```python
from build123d import *

# Parameters (mm, degrees)
SKETCH1_R             = 2
BOSS_EXTRUDE1_DEPTH   = 15
BOSS_EXTRUDE1_2_DEPTH = 15
SKETCH2_W             = 34.599574116
SKETCH2_H             = 26.046082642
BOSS_EXTRUDE2_DEPTH   = 2


with BuildPart() as part:
    # Sketch1 → Boss-Extrude1 (new body)
    with BuildSketch(Plane.XY):
        Circle(SKETCH1_R)
    extrude(amount=BOSS_EXTRUDE1_DEPTH)



with BuildPart() as body_2:
    # Sketch1 → Boss-Extrude1 2 (new body)
    with BuildSketch(Plane.XY):
        with Locations((28.8, -20.2)):
            Circle(SKETCH1_R)
    extrude(amount=BOSS_EXTRUDE1_2_DEPTH)


with BuildPart() as part_1:
    add(part.part)

    add(body_2.part)  # Boss-Extrude2 merges body 2
    # Sketch2 → Boss-Extrude2 (add)
    with BuildSketch(Plane.XY):
        with Locations((14.329889414, -10.310331758)):
            Rectangle(SKETCH2_W, SKETCH2_H)
    extrude(amount=-BOSS_EXTRUDE2_DEPTH)


solid = part_1.part
```
Source: CAD feature listing. Evaluate the final solid. Frame: model axes, mm. A direction names the side the tool comes from. Give positions to 0.01 mm unless a question says otherwise; leave off trailing zeros. Loops run counter-clockwise (first coordinate to the right, second up) from the corner with the lowest first, then second, coordinate; pieces in that order, holes last. Notation, with made-up numbers: (-23, -1.75) -> (3, -1.75) arc R18 cw to (3, 28.25) -> close; hole circle Ø5 at (66, -1.75). An arc over 180 degrees is marked (long way). Use a Markdown table: item, result. Add a question column.
(1) Access query for faces 1 (the face through (0, 0, 15)), 2 (the face through (26.802, -20.112, 7.395)). Directions: +Z, -Z, +X, -X, +Y, -Y. A direction counts if a zero-diameter tool reaches every point of the face in a straight line with its end or side. Return the directions, or none.
(2) Section query B-B (x = 28.8). Output: boundary loops of the cut face in (y, z), then the cut area to 3 significant figures.
(3) First-contact query: pin 1 Ø8 at (y, z) = (-2.5, 2.5) entering from +X; pin 2 Ø8 at (x, y) = (14.5, -6) entering from +Z. Flat tips, straight axial feed; report the tip coordinate or a pass-through.
(4) Ray query, line 1 (Z direction, x = 2, y = -2); line 2 (Y direction, x = 0, z = 13.5); line 3 (X direction, y = -19.5, z = 11). Return the intervals inside material, ascending.
(5) Section query C-C (z = 11.75). Output: boundary loops of the cut face in (x, y), then the cut area to 3 significant figures.
(6) Section query D-D (y = -4.25). Output: boundary loops of the cut face in (x, z), then the cut area to 3 significant figures.
(7) Section query A-A (y = -20.2). Output: boundary loops of the cut face in (x, z).
Checked values:
| question | item | result |
|---|---|---|
| 1 | face 1 | +Z, +X, -X, +Y, -Y |
| 1 | face 2 | +Z |
| 2 | outline | (-23.33, -2) -> (2.71, -2) -> (2.71, 0) -> (-18.2, 0) -> (-18.2, 15) -> (-22.2, 15) -> (-22.2, 0) -> (-23.33, 0) -> close |
| 2 | area | 112 mm^2 |
| 3 | pin 1 | x = 31.63 |
| 3 | pin 2 | z = 0 |
| 4 | line 1 | -2 to 0 |
| 4 | line 2 | -2 to 2 |
| 4 | line 3 | 26.93 to 30.67 |
| 5 | outline | circle Ø4 at (0, 0); circle Ø4 at (28.8, -20.2) |
| 5 | area | 25.1 mm^2 |
| 6 | outline | (-2.97, -2) -> (31.63, -2) -> (31.63, 0) -> (-2.97, 0) -> close |
| 6 | area | 69.2 mm^2 |
| 7 | outline | (-2.97, -2) -> (31.63, -2) -> (31.63, 0) -> (30.8, 0) -> (30.8, 15) -> (26.8, 15) -> (26.8, 0) -> (-2.97, 0) -> close |
